Answer from the drawing. Dimensions are ordinates in mm from the lowest x, y and z of the part. A direction names the side the tool comes from. Round coordinates to 2 decimals unless told otherwise and drop trailing zeros. Order: outer loops, then holes, each group sorted by start corner. A loop starts at its lowest first (then second) coordinate and runs counter-clockwise, first axis right, second up.
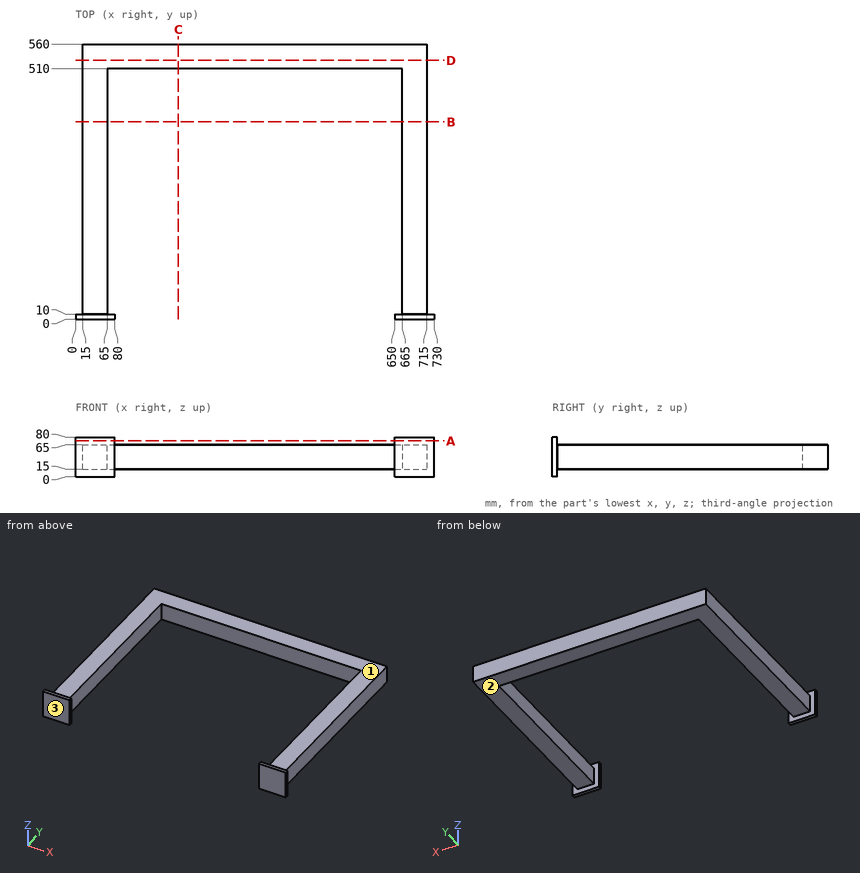
Q1. Straight lines are drawn through the part: probe 1 along X at (y, z) = (489, 53.5); probe 2 along Y at (x, z) = (651, 59); probe 3 along Y at (x, z) = (427.5, 22). For each, find the intervals that lie inside material, in ascending order.
Outcome:
probe 1: x = 15 to 65, 665 to 715
probe 2: y = 0 to 10, 510 to 560
probe 3: y = 510 to 560
Q2. A cutting plane is placed at D-D, the plane y = 526.5. Give the vertices of the cut face in (x, z).
Outcome:
outline: (15, 15) - (715, 15) - (715, 65) - (15, 65) - close
Q3. A cutting plane is placed at B-B, the plane y = 401.5. Give the vertices of the cut face in (x, z).
Outcome:
outline: (15, 15) - (65, 15) - (65, 65) - (15, 65) - close; (665, 15) - (715, 15) - (715, 65) - (665, 65) - close
Q4. Flat-ended cylindrical pins translate along their axes: pin 1 (5 mm diameter, centred on x = 255, z = 52, fed in from -Y); pin 2 (3 mm diameter, centred on y = 130.5, z = 20, fed in from -X); pin 3 (4 mm diameter, centred on y = 292.5, z = 32, fed in from +X). Find the tip coordinate at first contact, or state that the pin passes through.
Outcome:
pin 1: stops at y = 510
pin 2: stops at x = 15
pin 3: stops at x = 715
Q5. A cutting plane is placed at C-C, the plane x = 209.5. Give the vertices of the cut face in (y, z), plus the area to 3 significant figures.
Outcome:
outline: (510, 15) - (560, 15) - (560, 65) - (510, 65) - close
area: 2,500 mm2
Q6. A cutting plane is placed at A-A, the plane z = 72.5. Give the vertices of the cut face in (x, y), plus the area to 3 significant figures.
Outcome:
outline: (0, 0) - (80, 0) - (80, 10) - (0, 10) - close; (650, 0) - (730, 0) - (730, 10) - (650, 10) - close
area: 1,600 mm2
Q7. For the marked faces 1, 2 and 3, determine the directions among +Z, -Z, +X, -X, +Y, -Y from which every point of the face is accessible in a straight line to the end or side of a thin tool.
Outcome:
face 1: +Z, +X, -X, +Y
face 2: -Z, +X, -X, +Y
face 3: +Z, -Z, +X, -X, -Y
